Study the drawing (mm; zero at the part's minimum x, y, z) and answer. A direction names the side the tool comes from. Coordinates: 2 decimals unless noted, no trailing zeros. Order: outer loops, then holes, each group sorted by start corner. A loop starts at its lowest first (then second) coordinate and runs counter-clockwise, first axis right, second up.
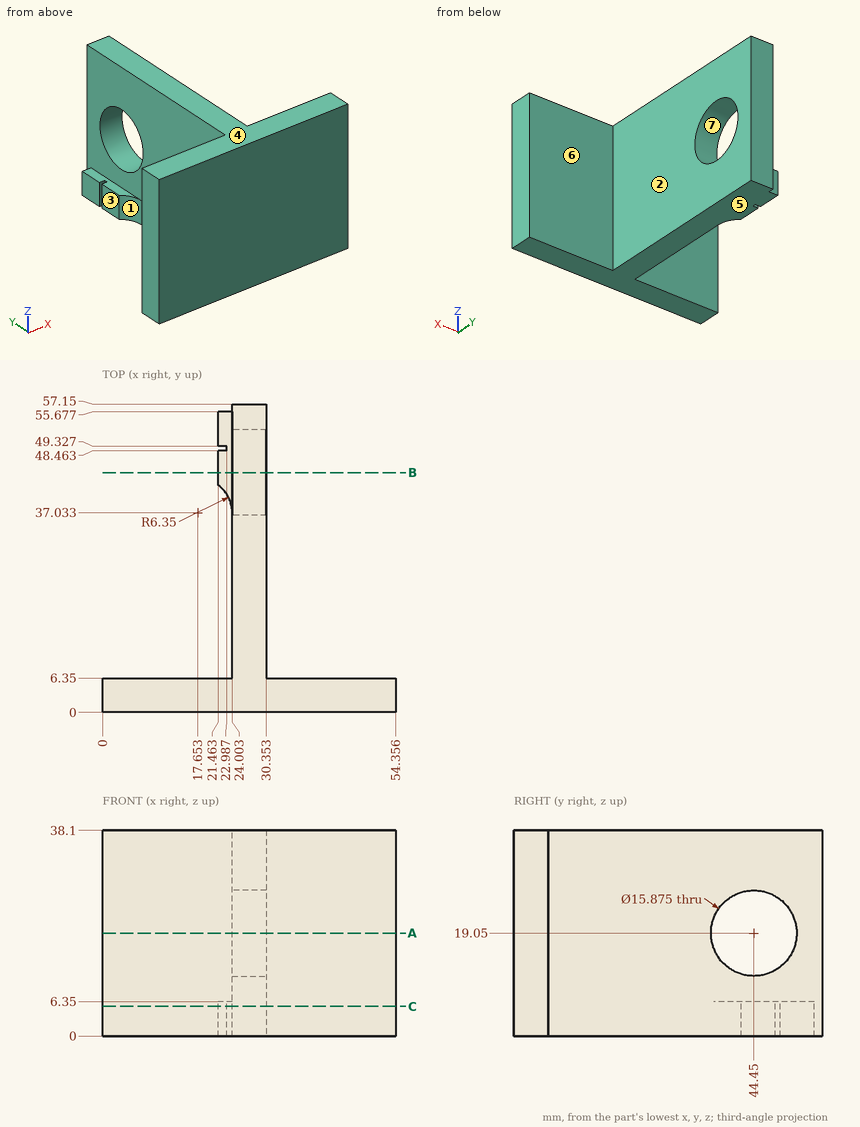
1) Flat-ended cylindrical pins translate along their axes: pin 1 Ø4 at (x, y) = (21.5, 48.5) entering from +Z; pin 2 Ø0.5 at (x, z) = (22, 4.5) entering from +Y; pin 3 Ø14.5 at (y, z) = (44.45, 19.05) entering from +X; pin 4 Ø1.9 at (y, z) = (51.5, 2.5) entering from -X. Find the tip coordinate at first contact, or state that the pin passes through.
A:
pin 1: stops at z = 6.35
pin 2: stops at y = 55.68
pin 3: passes through
pin 4: stops at x = 21.46
2) Determine the mould class of the marked faces 5, 6 and 7 for opening direction Y: pulls with the +Y half, pulls with the -Y half, needs draft (parallel to the pull), parting line crosses it, or undercut.
A:
face 5: needs draft
face 6: pulls with the +Y half
face 7: undercut
3) A cutting plane is placed at B-B, the plane y = 44.45. Determine the outline of the cut face in (x, z).
A:
outline: (21.46, 0) - (30.35, 0) - (30.35, 11.11) - (24, 11.11) - (24, 6.35) - (21.46, 6.35) - close; (24, 26.99) - (30.35, 26.99) - (30.35, 38.1) - (24, 38.1) - close
4) A cutting plane is placed at C-C, the plane z = 5.5. Determine the outline of the cut face in (x, y), and give its area (3 significant figures).
A:
outline: (0, 0) - (54.36, 0) - (54.36, 6.35) - (30.35, 6.35) - (30.35, 57.15) - (24, 57.15) - (24, 55.68) - (21.46, 55.68) - (21.46, 49.33) - (22.99, 49.33) - (22.99, 48.46) - (21.46, 48.46) - (21.46, 42.11) arc R6.35 cw to (24, 37.03) - (24, 6.35) - (0, 6.35) - close
area: 705 mm2
5) Straight lines are drawn through the part: line 1 (Z direction, x = 27.25, y = 44.45); line 2 (Y direction, x = 25, z = 19); line 3 (X direction, y = 35.5, z = 29). For each, find the intervals that lie inside material, in ascending order.
A:
line 1: z = 0 to 11.11, 26.99 to 38.1
line 2: y = 0 to 36.51, 52.39 to 57.15
line 3: x = 24 to 30.35
6) A cutting plane is placed at A-A, the plane z = 19.05. Determine the outline of the cut face in (x, y).
A:
outline: (0, 0) - (54.36, 0) - (54.36, 6.35) - (30.35, 6.35) - (30.35, 36.51) - (24, 36.51) - (24, 6.35) - (0, 6.35) - close; (24, 52.39) - (30.35, 52.39) - (30.35, 57.15) - (24, 57.15) - close
7) Which of the six approach directions +Z, -Z, +X, -X, +Y, -Y give full straight-line access (tool end or side, diameter ignored) to the marked faces 1, 2, 3 and 4?
A:
face 1: +Z, -Z, -X
face 2: +Z, -Z, +X, +Y
face 3: +Z, -Z, -X, +Y
face 4: +Z, +X, -X, +Y, -Y
